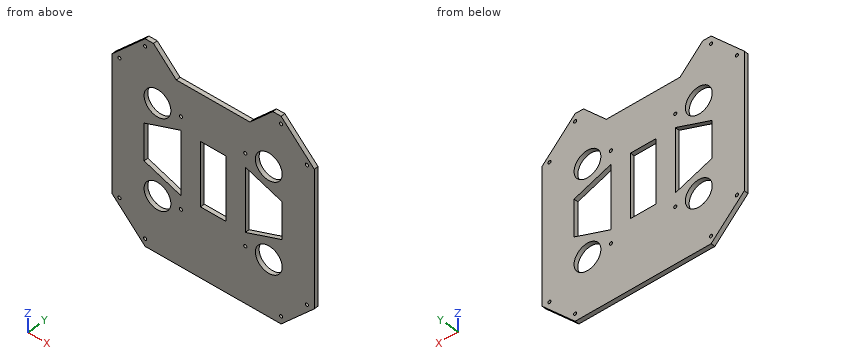
```python
from build123d import *

# Parameters (mm, degrees)
SKETCH1_R           = 40.4
SKETCH1_R_2         = 4.7625
BOSS_EXTRUDE1_DEPTH = 12.7
CUT_EXTRUDE1_DEPTH  = 5000
SKETCH3_R           = 4.7625
CUT_EXTRUDE2_DEPTH  = 5000
CUT_EXTRUDE3_DEPTH  = 20
SKETCH5_W           = 38.1
SKETCH5_H           = 192.02128445
CUT_EXTRUDE4_DEPTH  = 78.232


with BuildPart() as part:
    # Sketch1 → Boss-Extrude1 (new body)
    with BuildSketch(Plane(origin=(0, 0, 0), x_dir=(1, 0, 0), z_dir=(0, 1, 0))):
        Polygon((205, 0), (305, 100), (305, 510), (205, 610), (-205, 610), (-305, 510), (-305, 100), (-205, 0), align=None)
        with Locations((-167.82128445, 168.589357775)):
            Circle(SKETCH1_R, mode=Mode.SUBTRACT)
        with Locations((-97, 168.589357775)):
            Circle(SKETCH1_R_2, mode=Mode.SUBTRACT)
        with Locations((97, 168.589357775)):
            Circle(SKETCH1_R_2, mode=Mode.SUBTRACT)
        with Locations((167.82128445, 168.589357775)):
            Circle(SKETCH1_R, mode=Mode.SUBTRACT)
        with Locations((-167.82128445, 441.410642225)):
            Circle(SKETCH1_R, mode=Mode.SUBTRACT)
        with Locations((-97, 441.410642225)):
            Circle(SKETCH1_R_2, mode=Mode.SUBTRACT)
        with Locations((97, 441.410642225)):
            Circle(SKETCH1_R_2, mode=Mode.SUBTRACT)
        with Locations((167.82128445, 441.410642225)):
            Circle(SKETCH1_R, mode=Mode.SUBTRACT)
    extrude(amount=BOSS_EXTRUDE1_DEPTH)

    # Sketch2 → Cut-Extrude1 (cut)
    with BuildSketch(Plane(origin=(0, 12.7, 0), x_dir=(1, 0, 0), z_dir=(0, 1, 0))):
        Polygon((-111, 69), (-180, 0), (180, 0), (111, 69), align=None)
    extrude(amount=-CUT_EXTRUDE1_DEPTH, mode=Mode.SUBTRACT)

    # Sketch3 → Cut-Extrude2 (cut)
    with BuildSketch(Plane(origin=(0, 12.7, 0), x_dir=(1, 0, 0), z_dir=(0, 1, 0))):
        with Locations((-205, 22.45771137)):
            Circle(SKETCH3_R)
        with Locations((205, 22.45771137)):
            Circle(SKETCH3_R)
        with Locations((-282.54228863, 100)):
            Circle(SKETCH3_R)
        with Locations((282.54228863, 100)):
            Circle(SKETCH3_R)
        with Locations((282.54228863, 510)):
            Circle(SKETCH3_R)
        with Locations((205, 587.54228863)):
            Circle(SKETCH3_R)
        with Locations((-205, 587.54228863)):
            Circle(SKETCH3_R)
        with Locations((-282.54228863, 510)):
            Circle(SKETCH3_R)
    extrude(amount=-CUT_EXTRUDE2_DEPTH, mode=Mode.SUBTRACT)

    # Sketch4 → Cut-Extrude3 (cut)
    with BuildSketch(Plane(origin=(0, 12.7, 0), x_dir=(1, 0, 0), z_dir=(0, 1, 0))):
        Polygon((-208.22128445, 360.529405268), (-97, 401.010642225), (-97, 208.989357775), (-208.22128445, 249.470594732), align=None)
        Polygon((208.22128445, 249.470594732), (208.22128445, 360.529405268), (97, 401.010642225), (97, 208.989357775), align=None)
    extrude(amount=-CUT_EXTRUDE3_DEPTH, mode=Mode.SUBTRACT)

    # Sketch5 → Cut-Extrude4 (cut)
    with BuildSketch(Plane(origin=(0, 12.7, 0), x_dir=(1, 0, 0), z_dir=(0, 1, 0))):
        with Locations((-19.05, 305)):
            Rectangle(SKETCH5_W, SKETCH5_H)
        with Locations((19.05, 305)):
            Rectangle(SKETCH5_W, SKETCH5_H)
    extrude(amount=-CUT_EXTRUDE4_DEPTH, mode=Mode.SUBTRACT)


solid = part.part
```
The model under review builds one solid part; all positions refer to its coordinate system, in mm. Round coordinates to 2 decimals unless told otherwise and drop trailing zeros. Loops run counter-clockwise (first coordinate to the right, second up) from the corner with the lowest first, then second, coordinate; pieces in that order, holes last.
1) Consider section B-B on z = -314.5. State the section outline as (x, y) points, then the cut area to 3 significant figures.
Values follow:
outline: (-305, 0) - (-208.22, 0) - (-208.22, 12.7) - (-305, 12.7) - close; (-97, 0) - (-38.1, 0) - (-38.1, 12.7) - (-97, 12.7) - close; (38.1, 0) - (97, 0) - (97, 12.7) - (38.1, 12.7) - close; (208.22, 0) - (305, 0) - (305, 12.7) - (208.22, 12.7) - close
area: 3,950 mm2
2) Wall thickness on line 1 along X through (y, z) = (7.25, -100); line 2 along X through (y, z) = (4.5, -303); line 3 along Z through (x, y) = (-171, 9.5): over which ranges is each line inside the solid? List them lowest first.
Values follow:
line 1: x = -305 to -287.3, -277.78 to 277.78, 287.3 to 305
line 2: x = -305 to -208.22, -97 to -38.1, 38.1 to 97, 208.22 to 305
line 3: z = -610 to -481.69, -401.14 to -374.08, -235.92 to -208.86, -128.31 to -9
3) Clearance check with flat-ended pins moving along their axes: P1, Ø2, axis at x = 168.5, y = 6, coming from the +Z side; P2, Ø3, axis at x = -210.5, y = 9, coming from the +Z side; P3, Ø4, axis at x = -17, y = 8, coming from the +Z side. State where each tip first meets the part, or that it passes through.
Values follow:
P1: stops at z = -10.5
P2: stops at z = -4
P3: stops at z = -69
4) Consider section C-C on x = 140. State the section outline as (y, z) points, then the cut area to 3 significant figures.
Values follow:
outline: (0, -610) - (12.7, -610) - (12.7, -470.7) - (0, -470.7) - close; (0, -412.12) - (12.7, -412.12) - (12.7, -385.36) - (0, -385.36) - close; (0, -224.64) - (12.7, -224.64) - (12.7, -197.88) - (0, -197.88) - close; (0, -139.3) - (12.7, -139.3) - (12.7, -40) - (0, -40) - close
area: 3,710 mm2
5) Consider section A-A on x = 21.5. State the section outline as (y, z) points, then the cut area to 3 significant figures.
Values follow:
outline: (0, -610) - (12.7, -610) - (12.7, -401.01) - (0, -401.01) - close; (0, -208.99) - (12.7, -208.99) - (12.7, -69) - (0, -69) - close
area: 4,430 mm2
6) Consider section D-D on z = -409.5. State the section outline as (x, y) points.
Values follow:
outline: (-305, 0) - (-192.6, 0) - (-192.6, 12.7) - (-305, 12.7) - close; (-143.04, 0) - (143.04, 0) - (143.04, 12.7) - (-143.04, 12.7) - close; (192.6, 0) - (305, 0) - (305, 12.7) - (192.6, 12.7) - close
